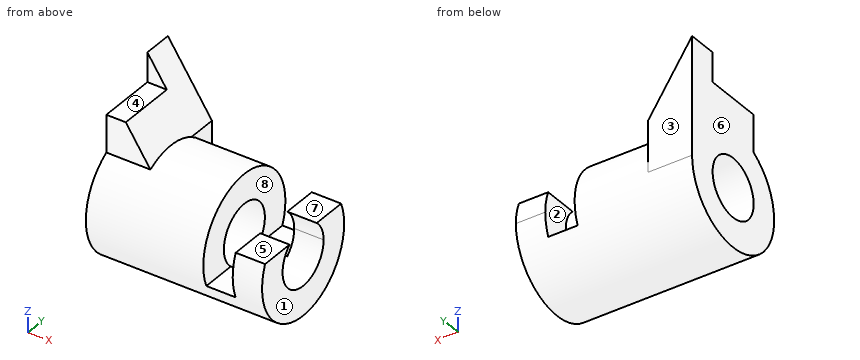
from build123d import *

# Parameters (mm, degrees)
F0_R          = 25.4
F0_R_2        = 12.7
F1_DEPTH      = 76.2
F3_DEPTH      = 25.4
F3_DEPTH_BACK = 25.4
F5_DEPTH      = 19.05
F6_W          = 25.4
F6_H          = 12.7
F7_DEPTH      = 25.4
F9_DEPTH      = 25.401
F9_DEPTH_BACK = 25.4


with BuildPart() as f1:
    # F0 (on Right) → F1 (new body)
    with BuildSketch(Plane.YZ):
        Circle(F0_R)
        Circle(F0_R_2, mode=Mode.SUBTRACT)
    extrude(amount=F1_DEPTH)

    # F2 (on Front) → F3 (cut, two sides)
    with BuildSketch(Plane.XZ) as f3_sk:
        Polygon((76.2, 25.4), (50.8, 25.4), (50.8, -9.525), (63.5, -9.525), (63.5, 9.525), (76.2, 9.525), align=None)
    extrude(amount=-F3_DEPTH, mode=Mode.SUBTRACT)
    extrude(f3_sk.sketch, amount=F3_DEPTH_BACK, mode=Mode.SUBTRACT)

    # F4 (on Right) → F5 (join)
    with BuildSketch(Plane.YZ):
        with BuildLine():
            Line((-12.7, 50.8), (-12.7, 0))
            ThreePointArc((-12.7, 0), (0, 12.7), (12.7, 0))
            Line((12.7, 0), (25.4, 0))
            Line((25.4, 0), (25.4, 50.8))
            Line((25.4, 50.8), (-12.7, 50.8))
        make_face()
    extrude(amount=F5_DEPTH)

    # F6 (on Right) → F7 (cut)
    with BuildSketch(Plane.YZ):
        with Locations((0, 44.45)):
            Rectangle(F6_W, F6_H)
    extrude(amount=F7_DEPTH, mode=Mode.SUBTRACT)

    # F8 (on Front) → F9 (cut, two sides)
    with BuildSketch(Plane.XZ) as f9_sk:
        Polygon((19.05, 50.8), (0, 50.8), (19.05, 21.9970452561), align=None)
    extrude(amount=F9_DEPTH, mode=Mode.SUBTRACT)
    extrude(f9_sk.sketch, amount=-F9_DEPTH_BACK, mode=Mode.SUBTRACT)


solid = f1.part
Model file for the job. Use its own axes, mm. Face numbers are marked on the shaded views. A direction names the side the tool comes from. Coordinates: 2 decimals unless noted, no trailing zeros. Order: outer loops, then holes, each group sorted by start corner. A loop starts at its lowest first (then second) coordinate and runs counter-clockwise, first axis right, second up. Notation, with made-up numbers: (63, -19.75) -> (117, -19.75) arc R33 cw to (117, 18.25) -> close; hole circle Ø5 at (78, 43.25). An arc over 180 degrees is marked (long way). Return JSON: item names as keys, results as strings. Group by question number.
Item 1: Flat gauge pins, fed straight in: P1, Ø12, axis at x = 26.5, y = 19, coming from the +Z side; P2, Ø6, axis at x = 11, y = -3, coming from the -Z side; P3, Ø6.5, axis at x = 2.5, y = -2.5, coming from the +Z side. Where does each tip first touch, or does it go through?
Item 2: Pull direction X, two halves, no side cores. Call the marked faces 6, 7 and 8: pulls with the +X half, pulls with the -X half, needs draft (parallel to the pull), parting line crosses it, or undercut.
Item 3: Saw through at A-A on y = 0. Write the cut outline in (x, z).
Item 4: Saw through at D-D on y = -7. Write the cut outline in (x, z).
Item 5: Tool access for the marked faces 1, 2, 3, 4 and 5: list every direction of +Z, -Z, +X, -X, +Y, -Y with a clear straight run to the whole face (end or side of a thin tool).
Item 6: Saw through at C-C on y = 18.5. Write the cut outline in (x, z) (3 decimals), then the cut area to 3 significant figures.
Item 7: Wall check: line 1 along Z through (x, y) = (32, 0); line 2 along X through (y, z) = (15, 5). Give the ranges that are in metal, low to high. Write a range as [from, to].
Item 8: Saw through at B-B on x = 15.5. Write the cut outline in (y, z).
Values found:
{
 "1": {"P1": "stops at z = 21.82", "P2": "stops at z = -25.4", "P3": "stops at z = 38.1"},
 "2": {"face 6": "pulls with the -X half", "face 7": "needs draft", "face 8": "undercut"},
 "3": {"outline": "(0, -25.4) -> (76.2, -25.4) -> (76.2, -12.7) -> (0, -12.7) -> close; (0, 12.7) -> (50.8, 12.7) -> (50.8, 25.4) -> (19.05, 25.4) -> (19.05, 22) -> (8.4, 38.1) -> (0, 38.1) -> close"},
 "4": {"outline": "(0, -24.42) -> (76.2, -24.42) -> (76.2, -10.6) -> (0, -10.6) -> close; (0, 10.6) -> (50.8, 10.6) -> (50.8, 24.42) -> (19.05, 24.42) -> (19.05, 22) -> (8.4, 38.1) -> (0, 38.1) -> close"},
 "5": {"face 1": "+Z, -Z, +X, +Y, -Y", "face 2": "+Z, +Y, -Y", "face 3": "+Z, -Z, +X, -X, +Y", "face 4": "+Z, +X, -X, -Y", "face 5": "+Z, +X, +Y, -Y"},
 "6": {"outline": "(0, -17.404) -> (76.2, -17.404) -> (76.2, 9.525) -> (63.5, 9.525) -> (63.5, -9.525) -> (50.8, -9.525) -> (50.8, 17.404) -> (19.05, 17.404) -> (19.05, 21.997) -> (0, 50.8) -> close", "area": "2,570 mm2"},
 "7": {"line 1": "z = [-25.4, -12.7], [12.7, 25.4]", "line 2": "x = [0, 50.8], [63.5, 76.2]"},
 "8": {"outline": "(-12.7, 22) arc R25.4 ccw (long way) to (25.4, 0) -> (25.4, 27.36) -> (-12.7, 27.36) -> close; hole circle Ø25.4 at (0, 0)"}
}
